For this review, take the finished solid that the model builds, in its own axes (mm). Face numbers are marked on the shaded views. A direction names the side the tool comes from. Round coordinates to 2 decimals unless told otherwise and drop trailing zeros. Order: outer loops, then holes, each group sorted by start corner. A loop starts at its lowest first (then second) coordinate and runs counter-clockwise, first axis right, second up. Notation, with made-up numbers: (46, 67.5) - (64, 67.5) arc R21 ccw to (64, 73.5) - close; hole circle Ø2 at (-13.75, -35). An arc over 180 degrees is marked (long way). One line per item, written item: value.
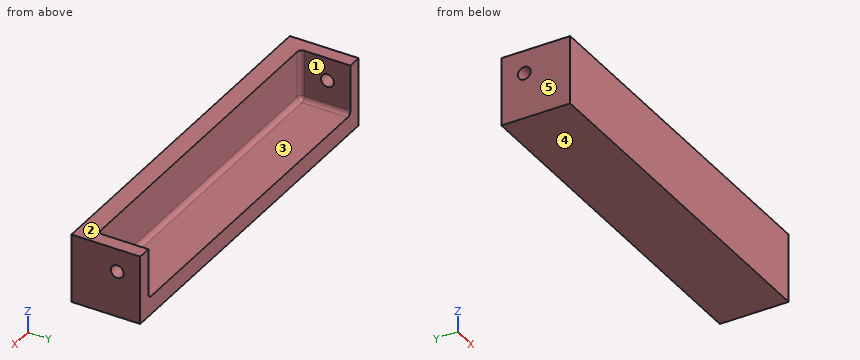
Autodesk Inventor part; units mm, degrees
ref_plane "YZ Plane" through (0, 0, 0) normal (1, 0, 0) x (0, 1, 0)
ref_plane "XZ Plane" through (0, 0, 0) normal (0, 1, 0) x (-1, 0, 0)
ref_plane "XY Plane" through (0, 0, 0) normal (0, 0, 1) x (1, 0, 0)
sketch "Sketch1" plane through (0, 0, 0) normal (0, 1, 0) x (-1, 0, 0)
  line L0 (39.5855, 7.487) -> (-40.4145, 7.487)
  line L1 (-40.4145, 7.487) -> (-40.4145, -7.513)
  line L2 (-40.4145, -7.513) -> (39.5855, -7.513)
  line L3 (39.5855, -7.513) -> (39.5855, 7.487)
  point P0 (0, 0)
  dimension "d0" = 80
  dimension "d1" = 15
extrude "Extrusion1" add sketch "Sketch1" along normal blind 15
sketch "Sketch2" plane through (0, 15, 0) normal (0, 1, 0) x (1, 0, 0)
  line L0 (-39.5855, -7.487) -> (40.4145, -7.487)
  line L1 (-36.5855, -7.487) -> (37.4145, -7.487)
  line L2 (37.4145, -7.487) -> (37.4145, 3.513)
  line L3 (37.4145, 3.513) -> (-36.5855, 3.513)
  line L4 (-36.5855, 3.513) -> (-36.5855, -7.487)
  line L5 (40.4145, 7.513) -> (-39.5855, 7.513)
  line L6 (-39.5855, 7.513) -> (-39.5855, -7.487)
  line L7 (40.4145, -7.487) -> (40.4145, 7.513)
  point P0 (0, 0)
  point P1 (37.4145, -7.487)
  dimension "d4" = 4
  dimension "d5" = 3
  dimension "d6" = 3
extrude "Extrusion2" cut sketch "Sketch2" against normal blind 11 contours L4 L3 L2 L0
sketch "Sketch3" plane through (-39.5855, 0, -7.513) normal (-1, 0, 0) x (0, 0, 1)
  circle A0 centre (10, 10) radius 1.4
  line L0 (15, 4) -> (4, 4)
  line L1 (4, 15) -> (4, 4)
  point P0 (7.513, 0)
  dimension "d9" = 2.8
  dimension "d10" = 6
  dimension "d11" = 6
extrude "Extrusion3" cut sketch "Sketch3" against normal through all
fillet "Fillet1" radius 1 1 edges at (0.4145, 4, -3.513)
fillet "Fillet2" radius 1 3 edges at (-36.5855, 10, -3.513) (-36.5855, 4.2929, -3.2201) (-36.5855, 4, 2.487)
fillet "Fillet3" radius 1 3 edges at (37.4145, 4, 2.487) (37.4145, 4.2929, -3.2201) (37.4145, 10, -3.513)
properties part number "leg_8"
Item 1: For P1, Ø3.5, axis at y = 10, z = 2.487, coming from the -X side; P2, Ø5, axis at x = 4, z = 1, coming from the +Y side; P3, Ø6, axis at x = 27, y = 9.5, coming from the +Z side; P4, Ø2, axis at y = 10, z = 2.487, coming from the -X side, all flat-tipped, find the tip position at first contact; note any pin that passes through.
Returned:
P1: x = -39.59
P2: y = 4
P3: z = -3.51
P4: through
Item 2: Take a section at A-A (y = 7.75). Write out the cut boundary in (x, z).
Returned:
outline: (-39.59, -7.51) - (40.41, -7.51) - (40.41, 7.49) - (37.41, 7.49) - (37.41, -2.51) arc R1 cw to (36.41, -3.51) - (-35.59, -3.51) arc R1 cw to (-36.59, -2.51) - (-36.59, 7.49) - (-39.59, 7.49) - close
Item 3: Take a section at B-B (z = 5.5). Write out the cut boundary in (x, y).
Returned:
outline: (-39.59, 0) - (40.41, 0) - (40.41, 15) - (37.41, 15) - (37.41, 5) arc R1 cw to (36.41, 4) - (-35.59, 4) arc R1 cw to (-36.59, 5) - (-36.59, 15) - (-39.59, 15) - close
Item 4: Take a section at C-C (x = -9). Write out the cut boundary in (y, z), plus the area to 3 significant figures.
Returned:
outline: (0, -7.51) - (15, -7.51) - (15, -3.51) - (5, -3.51) arc R1 cw to (4, -2.51) - (4, 7.49) - (0, 7.49) - close
area: 104 mm^2
Item 5: The part is to be moulded in two halves that separate along X. For the marked faces 3, 4 and 5, say which applies: +X half, -X half, draft (parallel to the pull), parting line (faces both ways), or undercut.
Returned:
face 3: undercut
face 4: draft
face 5: -X half
Item 6: Wall thickness on line 1 (X direction, y = 12, z = 4.75); line 2 (Z direction, x = -26, y = 7.5); line 3 (Y direction, x = -13.5, z = 2.5): over which ranges is each line inside the solid? List them lowest first.
Returned:
line 1: -39.59 to -36.59, 37.41 to 40.41
line 2: -7.51 to -3.51
line 3: 0 to 4
Item 7: Machinability: for the marked faces 1 and 2, which of the approach directions +Z, -Z, +X, -X, +Y, -Y give a long, thin tool a straight path to every point of the face, cutting with its end or side? Answer none if there is none.
Returned:
face 1: +Z, +Y
face 2: +Z, +X, -X, +Y, -Y
